Input: part model. Units: mm. Frame: model coordinates. Face numbers are marked on the shaded views. A direction names the side the tool comes from. Round coordinates to 2 decimals unless told otherwise and drop trailing zeros. Write each loop counter-clockwise with the first axis right and the second up, starting at its lowest first coordinate (ties: lowest second). Pieces come first, ordered by that corner, then holes. Notation, with made-up numbers: (39.25, -36.5) -> (53.25, -36.5) arc R17 ccw to (53.25, -21.5) -> close; hole circle Ø3 at (9.5, 72.25). An arc over 180 degrees is marked (long way). Use CSV: the item, a comma, the result in double quotes.
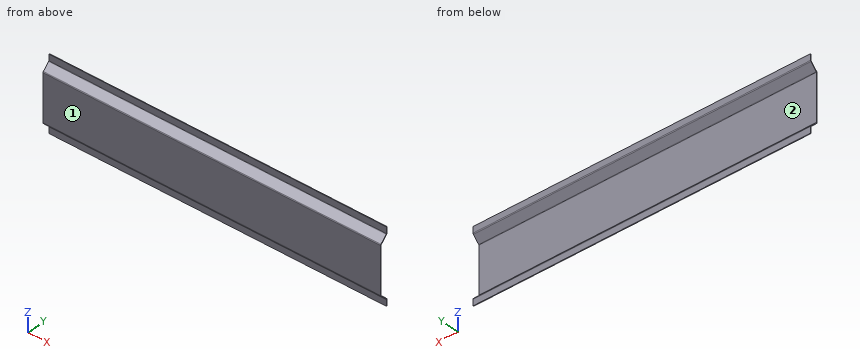
```python
from build123d import *

# Parameters (mm, degrees)
SM_BASE_FLANGE_1_DEPTH = 377


# Sheet-metal steps are written as plain solids
with BuildPart() as part:
    # Sketch 1 → Базовая кромка1 (new body)
    with BuildSketch(Plane(origin=(0, 0, 0), x_dir=(0, 0, -1), z_dir=(1, 0, 0))):
        with BuildLine():
            Line((0, -15), (-51.878679656, -15))
            ThreePointArc((-51.878679656, -15), (-52.452704805, -14.885819299), (-52.939339828, -14.560660172))
            Line((-52.939339828, -14.560660172), (-66.621320344, -0.878679656))
            ThreePointArc((-66.621320344, -0.878679656), (-67.59459039, -0.228361402), (-68.742640687, 0))
            Line((-68.742640687, 0), (-82.5, 0))
            Line((-82.5, 0), (-82.5, -1.5))
            Line((-82.5, -1.5), (-68.742640687, -1.5))
            ThreePointArc((-68.742640687, -1.5), (-68.168615539, -1.614180701), (-67.681980515, -1.939339828))
            Line((-67.681980515, -1.939339828), (-54, -15.621320344))
            ThreePointArc((-54, -15.621320344), (-53.026729954, -16.271638598), (-51.878679656, -16.5))
            Line((-51.878679656, -16.5), (0, -16.5))
            Line((0, -16.5), (0, -15))
        make_face()
    extrude(amount=-SM_BASE_FLANGE_1_DEPTH)

    # Зеркальное отражение1: part across plane


with BuildPart() as part_1:
    add(part.part)
    add(part.part.mirror(Plane(origin=(-494.133821974, -15, 0), x_dir=(1, 0, 0), z_dir=(0, 0, 1))))

    # Зеркальное отражение2: part across plane


with BuildPart() as part_2:
    add(part_1.part)
    add(part_1.part.mirror(Plane(origin=(0, -15.621320344, 54), x_dir=(0, 0, 1), z_dir=(1, 0, 0))))


solid = part_2.part
```
Item 1: Section query C-C on z = -37. Return the cut outline in (x, y), plus the area to 3 significant figures.
Worked answers:
outline,"(-377, -16.5) -> (377, -16.5) -> (377, -15) -> (-377, -15) -> close"
area,"1,130 mm²"
Item 2: Section query B-B on y = -9.5. Return the cut outline in (x, z), plus the area to 3 significant figures.
Worked answers:
outline,"(-377, -60.12) -> (377, -60.12) -> (377, -58) -> (-377, -58) -> close; (-377, 58) -> (377, 58) -> (377, 60.12) -> (-377, 60.12) -> close"
area,"3,200 mm²"
Item 3: Line query: line 1 (Y direction, x = -155, z = 8); line 2 (Z direction, x = -237, y = -0.25); line 3 (Z direction, x = -128, y = -2.25). Output: solid intervals per line, ascending.
Worked answers:
line 1,"y = -16.5 to -15"
line 2,"z = -82.5 to -67.54, 67.54 to 82.5"
line 3,"z = -67.37 to -65.25, 65.25 to 67.37"
Item 4: First-contact query: pin 1 Ø8 at (x, y) = (78.5, -3) entering from -Z; pin 2 Ø4 at (x, z) = (-247.5, -45.5) entering from +Y; pin 3 Ø5 at (x, y) = (-245.5, -14) entering from -Z; pin 4 Ø7 at (x, z) = (-52, -75) entering from -Y. Flat tips, straight axial feed; report the tip coordinate or a pass-through.
Worked answers:
pin 1,"stops at z = -82.5"
pin 2,"stops at y = -15"
pin 3,"stops at z = -58.12"
pin 4,"stops at y = -1.5"
Item 5: Set-up query: the marked faces 1 and 2. Return all of +Z, -Z, +X, -X, +Y, -Y with unobstructed straight access to the full face (end or side cutting, diameter ignored); none if empty.
Worked answers:
face 1,"+Z, -Z, +X, -X, -Y"
face 2,"+X, -X, +Y"
Item 6: Section query A-A on x = 82. Return the cut outline in (y, z), plus the area to 3 significant figures.
Worked answers:
outline,"(-16.5, -51.88) arc R3 ccw to (-15.62, -54) -> (-1.94, -67.68) arc R1.5 cw to (-1.5, -68.74) -> (-1.5, -82.5) -> (0, -82.5) -> (0, -68.74) arc R3 ccw to (-0.88, -66.62) -> (-14.56, -52.94) arc R1.5 cw to (-15, -51.88) -> (-15, 51.88) arc R1.5 cw to (-14.56, 52.94) -> (-0.88, 66.62) arc R3 ccw to (0, 68.74) -> (0, 82.5) -> (-1.5, 82.5) -> (-1.5, 68.74) arc R1.5 cw to (-1.94, 67.68) -> (-15.62, 54) arc R3 ccw to (-16.5, 51.88) -> close"
area,"266 mm²"
